Could you check a few things on this model? Use its own coordinates, in mm. A direction names the side the tool comes from. Round coordinates to 2 decimals unless told otherwise and drop trailing zeros. Write each loop counter-clockwise with the first axis right and the second up, starting at its lowest first coordinate (ties: lowest second). Pieces come first, ordered by that corner, then holes. Notation, with made-up numbers: (67.25, -22.75) -> (91.25, -22.75) arc R21 cw to (91.25, -13.75) -> close; hole circle Ø8 at (89.25, 48). An arc over 180 degrees is marked (long way). Answer in a Markdown table with one row per item. Add a question column.
Autodesk Inventor part; units mm, degrees
ref_plane "YZ Plane" through (0, 0, 0) normal (1, 0, 0) x (0, 1, 0)
ref_plane "XZ Plane" through (0, 0, 0) normal (0, 1, 0) x (-1, 0, 0)
ref_plane "XY Plane" through (0, 0, 0) normal (0, 0, 1) x (1, 0, 0)
sketch "Sketch1" plane through (0, 0, 0) normal (0, 0, 1) x (1, 0, 0)
  circle A0 centre (0, 0) radius 125
  dimension "d0" = 250
extrude "Extrusion1" add sketch "Sketch1" along normal blind 15
sketch "Sketch2" plane through (0, 0, 15) normal (0, 0, 1) x (1, 0, 0)
  circle A0 centre (0, 0) radius 25
  dimension "d3" = 50
extrude "Extrusion2" cut sketch "Sketch2" against normal blind 7
sketch "Sketch3" plane through (0, 0, 8) normal (0, 0, 1) x (1, 0, 0)
  circle A0 centre (0, 0) radius 12.5
  dimension "d6" = 25
extrude "Extrusion3" cut sketch "Sketch3" against normal through all
sketch "Sketch4" plane through (0, 0, 15) normal (0, 0, 1) x (1, 0, 0)
  circle A0 centre (29.5, -48.5) radius 1.6
  line L0 (0, 0) -> (147.2327, 0)
  line L1 (93, 0) -> (93, 59.5)
  circle A1 centre (29.5, 48.5) radius 1.6
  circle A2 centre (93, -59.5) radius 1.6
  circle A3 centre (93, 59.5) radius 1.6
  circle A4 centre (104, 0) radius 1.6
  dimension "d11" = 3.2
  dimension "d50" = 93
  dimension "d51" = 3.2
  dimension "d53" = 3.2
  dimension "d55" = 97
  dimension "d56" = 119
  dimension "d90" = 29.5
  dimension "d91" = 104
extrude "Extrusion4" cut sketch "Sketch4" against normal blind 8
sketch "Sketch5" plane through (0, 0, 15) normal (0, 0, 1) x (1, 0, 0)
  line L0 (-43.6176, 0) -> (7.6417, 0)
  circle A0 centre (-40, 44.5) radius 1.6
  circle A1 centre (-40, -44.5) radius 1.6
  line L1 (-71, 46.1) -> (-71, -32.5719)
  circle A2 centre (-102, 44.5) radius 1.6
  circle A3 centre (-102, -44.5) radius 1.6
  circle A4 centre (-113, 0) radius 1.6
  point P0 (0, 0)
  dimension "d60" = 3.2
  dimension "d61" = 89
  dimension "d62" = 62
  dimension "d63" = 40
  dimension "d64" = 3.2
  dimension "d65" = 11
extrude "Extrusion5" cut sketch "Sketch5" against normal blind 8
sketch "Sketch6" plane through (0, 0, 15) normal (0, 0, 1) x (1, 0, 0)
  circle A0 centre (-42, 85) radius 1.6
  line L0 (0, 131.4928) -> (0, 57.1829)
  line L1 (-43.3756, 85) -> (37.4091, 85)
  circle A1 centre (42, 85) radius 1.6
  circle A2 centre (0, 111) radius 1.6
  circle A3 centre (0, 59) radius 1.6
  point P0 (0, 0)
  dimension "d38" = 3.2
  dimension "d85" = 85
  dimension "d86" = 84
  dimension "d87" = 3.2
  dimension "d88" = 52
extrude "Extrusion6" cut sketch "Sketch6" against normal blind 8
sketch "Sketch9" plane through (0, 0, 15) normal (0, 0, 1) x (1, 0, 0)
  line L0 (0, -68.2489) -> (0, -119.1894)
  line L1 (-34.7906, -80) -> (35.8893, -80)
  circle A0 centre (-30, -60) radius 1.6
  circle A1 centre (30, -60) radius 1.6
  circle A2 centre (-30, -100) radius 1.6
  circle A3 centre (30, -100) radius 1.6
  point P0 (0, 0)
  point P1 (0.5493, -80)
  dimension "d77" = 80
  dimension "d78" = 3.2
  dimension "d79" = 60
  dimension "d89" = 40
extrude "Extrusion8" cut sketch "Sketch9" against normal blind 8
sketch "Sketch7" plane through (0, 0, 0) normal (0, 0, -1) x (-1, 0, 0)
  circle A0 centre (77.5, 42.5) radius 1.6
  circle A1 centre (0, 0) radius 12.5
  line L0 (0, 0) -> (77.5, 0)
  circle A2 centre (77.5, -42.5) radius 1.6
  line L1 (0, 0) -> (26.3155, 0)
  line L2 (77.5, 42.5) -> (77.5, -42.5)
  dimension "d66" = 3.2
  dimension "d67" = 85
  dimension "d75" = 0
  dimension "d76" = 77.5
extrude "Extrusion7" cut sketch "Sketch7" against normal blind 8 contours A0 | A2
pattern_circular "Circular Pattern1" count 4 over 360 about axis through (0, 0, 8) along (0, 0, -1) of "Extrusion7"
sketch "Sketch8" plane through (0, 0, 15) normal (0, 0, 1) x (1, 0, 0)
  point P0 (0, 0)
properties part number "base_board"
(1) Suppose I cut it at D-D, the plane y = 71. Please give me the cut outline in (x, z).
(2) I need wall thicknesses on L1, parallel to Y at x = 0, z = 12.75; L2, parallel to Y at x = -77.5, z = 5.5. Which ranges of each line are inside material? Lowest first, please.
(3) For P1, Ø3, axis at x = 38.5, z = 10, coming from the -Y side; P2, Ø1.6, axis at x = -112.5, y = -0.5, coming from the +Z side; P3, Ø2, axis at x = 63, z = 2, coming from the +Y side, each with a flat end and sliding along its axis, tell me the tip position at first contact or that it passes through.
(4) Suppose I cut it at C-C, the plane x = 20.5. Please give me the cut outline in (y, z), then the cut area to 3 significant figures.
(5) Suppose I cut it at B-B, the plane y = -5.5. Please give me the cut outline in (x, z), then the cut area to 3 significant figures.
(6) On a 3-axis mill with a long thin cutter (end or side, diameter ignored), from which of +Z, -Z, +X, -X, +Y, -Y can I reach the whole of each face in a straight line? I mean faces 4 (the face through (-2, -26, 0)), 5 (the face through (23.846, 7.509, 11.549)). Say none if no direction works.
(7) Suppose I cut it at A-A, the plane z = 12.75. State how many separate pieces and enclosed holes the cut face has, then the cut area to 3 significant figures.
(8) If we mould it in two halves opening along Y, with no side actions, what happens to faces 1 (the face through (-2, -26, 15)), 2 (the face through (-5.9, 11.5, 8)), 3 (the face through (-124.88, -5.5, 7.4))? For each: pulls with the +Y half, pulls with the -Y half, needs draft (parallel to the pull), parting line crosses it, or undercut.
Response:
| question | item | result |
|---|---|---|
| 1 | outline | (-102.88, 0) -> (102.88, 0) -> (102.88, 15) -> (-102.88, 15) -> close |
| 2 | L1 | -125 to -25, 25 to 57.4, 60.6 to 109.4, 112.6 to 125 |
| 2 | L2 | -98.08 to -44.1, -40.9 to 40.9, 44.1 to 98.08 |
| 3 | P1 | y = -119.4 |
| 3 | P2 | z = 7 |
| 3 | P3 | y = 108.54 |
| 4 | outline | (-123.31, 0) -> (123.31, 0) -> (123.31, 15) -> (14.31, 15) -> (14.31, 8) -> (-14.31, 8) -> (-14.31, 15) -> (-123.31, 15) -> close |
| 4 | area | 3,500 mm² |
| 5 | outline | (-124.88, 0) -> (-11.22, 0) -> (-11.22, 8) -> (-24.39, 8) -> (-24.39, 15) -> (-124.88, 15) -> close; (11.22, 0) -> (124.88, 0) -> (124.88, 15) -> (24.39, 15) -> (24.39, 8) -> (11.22, 8) -> close |
| 5 | area | 3,230 mm² |
| 6 | face 4 | -Z, +X, -X, +Y, -Y |
| 6 | face 5 | +Z |
| 7 | separate pieces | 1 |
| 7 | enclosed holes | 19 |
| 7 | area | 47,000 mm² |
| 8 | face 1 | needs draft |
| 8 | face 2 | undercut |
| 8 | face 3 | parting line crosses it |
